Design review of the part built by this model. Coordinates are the model's own, in mm. A direction names the side the tool comes from. Coordinates: 2 decimals unless noted, no trailing zeros. Write each loop counter-clockwise with the first axis right and the second up, starting at its lowest first coordinate (ties: lowest second). Pieces come first, ordered by that corner, then holes. Notation, with made-up numbers: M 24,-25.5 L 31,-25.5 A16 cw 31,-4.5 Z; hole C 47,82.25 d4. An arc over 180 degrees is marked long. Write item = value, one per line.
```python
from build123d import *

# Parameters (mm, degrees)
SKETCH1_W            = 26
SKETCH1_H            = 26
SKETCH1_R            = 10.4
BOSS_EXTRUDE2_DEPTH  = 60
SKETCH2_R            = 1.6
CUT_EXTRUDE1_DEPTH   = 67.670833203
CUT_EXTRUDE2_DEPTH   = 2
SKETCH4_R            = 3
CUT_EXTRUDE3_DEPTH   = 2
CUT_EXTRUDE5_DEPTH   = 63.753486055
SKETCH7_W            = 26
SKETCH7_H            = 26
BOSS_EXTRUDE3_DEPTH  = 20
SKETCH8_R            = 1.6
CUT_EXTRUDE6_DEPTH   = 57.177126928
SKETCH9_R            = 3
CUT_EXTRUDE7_DEPTH   = 2
CUT_EXTRUDE8_DEPTH   = 2
SKETCH11_OUTSIDE_W   = 50.774
SKETCH11_OUTSIDE_H   = 78.112
SKETCH11_OUTSIDE_R   = 13
SKETCH11_OUTSIDE_R_2 = 10.4
CUT_EXTRUDE9_DEPTH   = 20
SKETCH5_OUTSIDE_W    = 46.131
SKETCH5_OUTSIDE_H    = 63.995
CUT_EXTRUDE4_DEPTH   = 71.049051406
SKETCH13_R           = 13
BOSS_EXTRUDE4_DEPTH  = 7
FILLET1_R            = 2
SKETCH14_R           = 10.4
CUT_EXTRUDE10_DEPTH  = 71.049051406


with BuildPart() as part:
    # Sketch1 → Boss-Extrude2 (new body)
    with BuildSketch(Plane.XY):
        Rectangle(SKETCH1_W, SKETCH1_H)
        Circle(SKETCH1_R, mode=Mode.SUBTRACT)
    extrude(amount=BOSS_EXTRUDE2_DEPTH)

    # Sketch2 → Cut-Extrude1 (cut, through all)
    with BuildSketch(Plane.ZY.offset(13)):
        with Locations((30, 0)):
            Circle(SKETCH2_R)
    extrude(amount=-CUT_EXTRUDE1_DEPTH, mode=Mode.SUBTRACT)

    # Sketch3 → Cut-Extrude2 (cut)
    with BuildSketch(Plane.ZY.offset(13)):
        Polygon((33.348631561, 0), (31.674315781, 2.9), (28.325684219, 2.9), (26.651368439, 0), (28.325684219, -2.9), (31.674315781, -2.9), align=None)
    extrude(amount=-CUT_EXTRUDE2_DEPTH, mode=Mode.SUBTRACT)

    # Sketch4 → Cut-Extrude3 (cut)
    with BuildSketch(Plane(origin=(13, 0, 0), x_dir=(0, 0, -1), z_dir=(1, 0, 0))):
        with Locations((-30, 0)):
            Circle(SKETCH4_R)
    extrude(amount=-CUT_EXTRUDE3_DEPTH, mode=Mode.SUBTRACT)

    # Sketch6 → Cut-Extrude5 (cut, through all)
    with BuildSketch(Plane.XY.offset(60)):
        Polygon((-13, 13), (13, 13), (13, 10.267289883), align=None)
    extrude(amount=-CUT_EXTRUDE5_DEPTH, mode=Mode.SUBTRACT)

    # Sketch7 → Boss-Extrude3 (add)
    with BuildSketch(Plane(origin=(1.209385395, 11.506533414, 0), x_dir=(0.9945218953682742, -0.1045284632676464, 0), z_dir=(0.1045284632676464, 0.9945218953682742, 0))):
        with Locations((-1.216047028, -30)):
            Rectangle(SKETCH7_W, SKETCH7_H)
    extrude(amount=BOSS_EXTRUDE3_DEPTH)

    # Sketch8 → Cut-Extrude6 (cut, through all)
    with BuildSketch(Plane.XY.offset(43)):
        with Locations((1.080892313, 21.575121377)):
            Circle(SKETCH8_R)
    extrude(amount=-CUT_EXTRUDE6_DEPTH, mode=Mode.SUBTRACT)

    # Sketch9 → Cut-Extrude7 (cut)
    with BuildSketch(Plane.XY.offset(43)):
        with Locations((1.080892313, 21.575121377)):
            Circle(SKETCH9_R)
    extrude(amount=-CUT_EXTRUDE7_DEPTH, mode=Mode.SUBTRACT)

    # Sketch10 → Cut-Extrude8 (cut)
    with BuildSketch(Plane(origin=(0, 0, 17), x_dir=(-1, 0, 0), z_dir=(0, 0, -1))):
        Polygon((2.267739249, 21.575121377), (0.593423468, 24.475121377), (-2.755208093, 24.475121377), (-4.429523874, 21.575121377), (-2.755208093, 18.675121377), (0.593423468, 18.675121377), align=None)
    extrude(amount=-CUT_EXTRUDE8_DEPTH, mode=Mode.SUBTRACT)

    # Sketch11 outside → Cut-Extrude9 (cut)
    # profile 1 of 2: a face of its own
    with BuildSketch(Plane(origin=(3.29995466, 31.396971322, 0), x_dir=(0.9945218953682742, -0.10452846326764643, 0), z_dir=(0.10452846326764643, 0.9945218953682742, 0))):
        with Locations((-0.035, -30)):
            Rectangle(SKETCH11_OUTSIDE_W, SKETCH11_OUTSIDE_H)
        with Locations(Location((-1.216047028, -30, 0), (0, 0, 180))):
            Circle(SKETCH11_OUTSIDE_R, mode=Mode.SUBTRACT)
    # profile 2 of 2: a face of its own
    with BuildSketch(Plane(origin=(3.29995466, 31.396971322, 0), x_dir=(0.9945218953682742, -0.10452846326764643, 0), z_dir=(0.10452846326764643, 0.9945218953682742, 0))):
        with Locations(Location((-1.216047028, -30, 0), (0, 0, 180))):
            Circle(SKETCH11_OUTSIDE_R_2)
    extrude(amount=-CUT_EXTRUDE9_DEPTH, mode=Mode.SUBTRACT)

    # Sketch5 outside → Cut-Extrude4 (cut, through all)
    with BuildSketch(Plane.XY.offset(60)):
        with Locations((1.0095, 9.9415)):
            Rectangle(SKETCH5_OUTSIDE_W, SKETCH5_OUTSIDE_H)
        with BuildLine():
            Line((-6.92820323, -11), (-6.92820323, -13))
            Line((-6.92820323, -13), (6.92820323, -13))
            Line((6.92820323, -13), (6.92820323, -11))
            ThreePointArc((6.92820323, -11), (12.999577974, -0.104749706), (7.104566567, 10.886924906))
            Line((7.104566567, 10.886924906), (13, 10.267289883))
            Line((13, 10.267289883), (15.291712761, 31.831368542))
            Line((15.291712761, 31.831368542), (-10.708287239, 34.594506849))
            Line((-10.708287239, 34.594506849), (-13, 13))
            Line((-13, 13), (-4.685795776, 12.126141923))
            ThreePointArc((-4.685795776, 12.126141923), (-12.939314251, 1.254650033), (-6.92820323, -11))
        make_face(mode=Mode.SUBTRACT)
    extrude(amount=-CUT_EXTRUDE4_DEPTH, mode=Mode.SUBTRACT)

    # Sketch13 → Boss-Extrude4 (add)
    with BuildSketch(Plane(origin=(1.209385395, 11.506533414, 0), x_dir=(0.9945218953682741, -0.10452846326764687, 0), z_dir=(-0.10452846326764687, -0.9945218953682741, 0))):
        with Locations(Location((-1.216047028, 30, 0), (0, 0, 180))):
            Circle(SKETCH13_R)
    extrude(amount=BOSS_EXTRUDE4_DEPTH)

    # Fillet1
    # the kernel refuses this fillet: 2 mm, written as the material it adds along each edge
    with BuildSketch(Plane(origin=(-11.625930527, 5.817021522, 16.479857089), x_dir=(-0.36199929686843824, -0.9321783676243277, 0), z_dir=(0, 0, 1))) as fillet1_piece_1_section:
        with BuildLine():
            CenterArc((2.614603278, -1.991261329), FILLET1_R, 95.358010672, 99.865019887)
            Line((0.684781224, -2.516415439), (0, 0))
            ThreePointArc((0, 0), (1.213922951, -0.056801359), (2.427845901, 0))
        make_face()
    fillet1_piece_1 = extrude(amount=27.040285822, mode=Mode.PRIVATE)
    fillet1_piece_1 = fillet1_piece_1 & Plane(origin=(-0.793541371, 4.083603133, 30), x_dir=(-0.9945218953682741, 0.10452846326764687, 0), z_dir=(0.10452846326764687, 0.9945218953682741, 0)) * Cylinder(13, 65, mode=Mode.PRIVATE)
    add(fillet1_piece_1)

    # Sketch14 → Cut-Extrude10 (cut, through all)
    with BuildSketch(Plane.XY.offset(60)):
        Circle(SKETCH14_R)
    extrude(amount=-CUT_EXTRUDE10_DEPTH, mode=Mode.SUBTRACT)


solid = part.part
```
Q1. Machinability: for faces 4 (the flat face through (-12.014, -1.43, 27.477)), 5 (the flat face through (11, -1.3, 28.7)), 6 (the flat face through (3.58, 23.05, 18.02)), 7 (the cylindrical face through (2.7, 24.1, 42)), which of the approach directions +Z, -Z, +X, -X, +Y, -Y give a long, thin tool a straight path to every point of the face, cutting with its end or side? Answer none if there is none.
Check result:
face_4 = -X
face_5 = +X
face_6 = -Z
face_7 = +Z
Q2. For P1, Ø5, axis at x = 10, z = 39, coming from the -Y side; P2, Ø1.7, axis at x = 0, y = 20.5, coming from the -Z side; P3, Ø8, axis at x = 1.08, y = 21.58, coming from the +Z side; P4, Ø1.9, axis at y = 0, z = 30, coming from the -X side, all flat-tipped, find the tip position at first contact; note any pin that passes through.
Check result:
P1 = -10.62
P2 = 19
P3 = 43
P4 = through
Q3. The part is to be moulded in two halves that separate along Y. For faces 1 (the flat face through (3, 22, 19)), 2 (the flat face through (0, -13, 30)), 3 (the flat face through (1, -11, 60)), say which applies: +Y half, -Y half, draft (parallel to the pull), parting line (faces both ways), or undercut.
Check result:
face_1 = undercut
face_2 = -Y half
face_3 = draft
Q4. Wall thickness on line 1 (X direction, y = 0, z = 37); line 2 (Z direction, x = 10.6, y = 0); line 3 (Y direction, x = -8.5, z = 16): over which ranges is each line inside the solid? List them lowest first.
Check result:
line_1 = -13 to -10.4, 10.4 to 13
line_2 = 0 to 28.4, 31.6 to 60
line_3 = -9.84 to -5.99, 5.99 to 9.84
Q5. Consider section C-C, the plane z = 39. State the section outline as (x, y) points, and give its area (3 significant figures).
Check result:
outline = M -9.75,8.6 A13 ccw -6.93,-11 L -6.93,-13 L 6.93,-13 L 6.93,-11 A13 ccw 9.18,9.21 L 11.42,30.54 L 7.27,30.98 L 5.18,11.09 L -5.18,12.18 L -3.09,32.07 L -7.24,32.5 Z; hole C 0,0 d20.8
area = 365 mm²
Q6. Consider section A-A, the plane z = 50. State the section outline as (x, y) points, and give its area (3 significant figures).
Check result:
outline = M -6.93,-13 L 6.93,-13 L 6.93,-11 A13 ccw 7.1,10.89 L -4.69,12.13 A13 ccw -6.93,-11 Z; hole C 0,0 d20.8
area = 189 mm²
